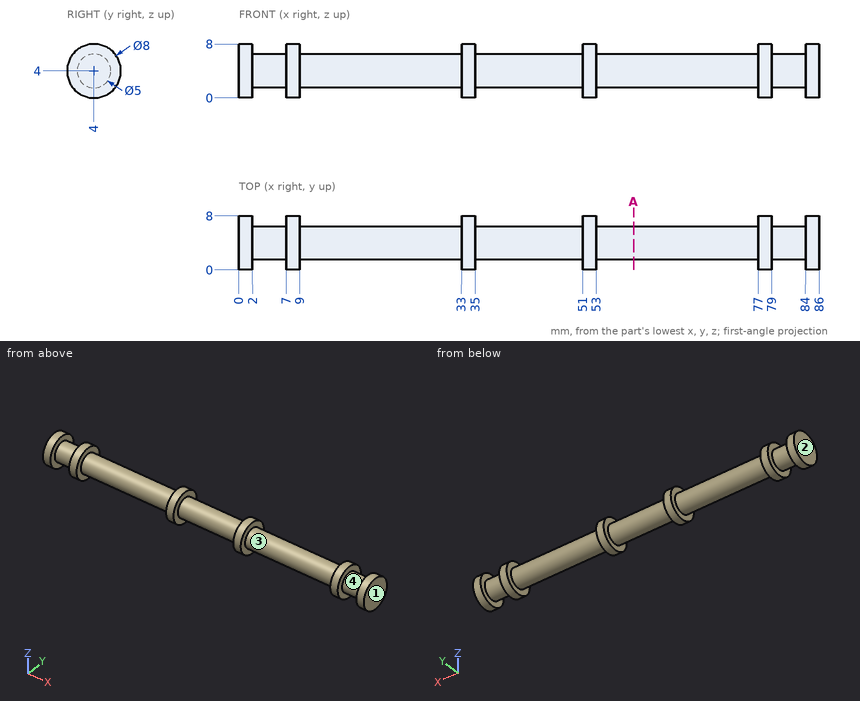
Geometry: see drawing. Coordinates: mm, zero at the bounding-box minimum. Round coordinates to 2 decimals unless told otherwise and drop trailing zeros. Loops run counter-clockwise (first coordinate to the right, second up) from the corner with the lowest first, then second, coordinate; pieces in that order, holes last. Notation, with made-up numbers: (34, -36) - (70, -36) arc R15 ccw to (70, -11) - close; hole circle Ø3 at (40.5, 40.25). An arc over 180 degrees is marked (long way). Write item = value, one per line. Start each with the question number.
(1) Section query A-A, the plane x = 58.5. Output: boundary loops of the cut face in (y, z).
(2) Pull-direction query (X, two-part tool) for the marked faces 1, 2, 3 and 4; classes: +X half, -X half, draft (parallel to the pull), parting line (faces both ways), or undercut.
(3) Pin query (flat end, axial travel): pin 1 (4 mm diameter, centred on x = 17.5, z = 7, fed in from -Y); pin 2 (3 mm diameter, centred on x = 17.5, y = 2.5, fed in from -Z); pin 3 (1.5 mm diameter, centred on x = 19.5, z = 6, fed in from -Y). Return the tip coordinate at first contact, or that it passes through.
(4) Ray query, line 1 along X through (y, z) = (3, 1.25); line 2 along Z through (x, y) = (44, 4); line 3 along Y through (x, z) = (75.5, 6.25). Return the intervals inside material, ascending. Write a range as from..to.
Conclusion:
q1.outline = circle Ø5 at (4, 4)
q2.face_1 = +X half
q2.face_2 = -X half
q2.face_3 = undercut
q2.face_4 = undercut
q3.pin_1 = 1.71
q3.pin_2 = 1.5
q3.pin_3 = 1.83
q4.line_1 = 0..2, 7..9, 33..35, 51..53, 77..79, 84..86
q4.line_2 = 1.5..6.5
q4.line_3 = 2.91..5.09
